```python
from build123d import *

# Parameters (mm, degrees)
BOSS_EXTRUDE2_DEPTH = 57.15
BOSS_EXTRUDE3_DEPTH = 44
CUT_EXTRUDE1_DEPTH  = 44
FILLET1_R           = 10
SKETCH6_W           = 120
SKETCH6_H           = 460.0000000000001
BOSS_EXTRUDE4_DEPTH = 10


with BuildPart() as part:
    # Sketch1 → Boss-Extrude2 (new body)
    with BuildSketch(Plane.XY):
        Polygon((0, 0), (0, 446.2018372120283), (-775, 446.2018372120282), (-774.9999999999995, -1585.7981627879717), (0, -1585.7981627879717), align=None)
    extrude(amount=BOSS_EXTRUDE2_DEPTH)

    # Sketch4 → Boss-Extrude3 (add)
    with BuildSketch(Plane.XY.offset(57.15)):
        Polygon((-79.99999999999993, -603.7981627879718), (-49.999999999999936, -603.7981627879718), (-49.999999999999915, -785.7981627879718), (-79.9999999999999, -785.7981627879718), align=None)
    extrude(amount=BOSS_EXTRUDE3_DEPTH)

    # Sketch5 → Cut-Extrude1 (cut)
    with BuildSketch(Plane.ZY.offset(80.00000000000003)):
        Polygon((83.14999999999999, -624.7981627879717), (57.150000000000006, -624.7981627879717), (57.15, -764.7981627879717), (83.15, -764.7981627879717), align=None)
    extrude(amount=-CUT_EXTRUDE1_DEPTH, mode=Mode.SUBTRACT)

    # Fillet1
    # the kernel refuses this fillet: 10 mm, written as the material it takes off along each edge
    with BuildSketch(Plane(origin=(-69.99999999999993, -613.7981627879718, 91.15), x_dir=(-1, -1.6e-16, 0), z_dir=(0, 1, 0))) as fillet1_piece_1_section:
        Polygon((0, 0), (FILLET1_R, 0), (FILLET1_R, FILLET1_R), (0, FILLET1_R), align=None)
    fillet1_piece_1 = extrude(amount=FILLET1_R, mode=Mode.PRIVATE)
    fillet1_piece_1 = fillet1_piece_1 - Plane(origin=(-69.99999999999993, -613.7981627879718, 91.15), x_dir=(0.7071067811865475, 0, -0.7071067811865475), z_dir=(0, 1, 0)) * Sphere(FILLET1_R, mode=Mode.PRIVATE)
    add(fillet1_piece_1, mode=Mode.SUBTRACT)
    with BuildSketch(Plane(origin=(-69.9999999999999, -775.7981627879718, 91.15), x_dir=(0, 0, 1), z_dir=(-1, -1.6e-16, 0))) as fillet1_piece_2_section:
        Polygon((0, 0), (FILLET1_R, 0), (FILLET1_R, -FILLET1_R), (0, -FILLET1_R), align=None)
    fillet1_piece_2 = extrude(amount=FILLET1_R, mode=Mode.PRIVATE)
    fillet1_piece_2 = fillet1_piece_2 - Plane(origin=(-69.9999999999999, -775.7981627879718, 91.15), x_dir=(0, 0.7071067811865475, -0.7071067811865475), z_dir=(-1, -1.6e-16, 0)) * Sphere(FILLET1_R, mode=Mode.PRIVATE)
    add(fillet1_piece_2, mode=Mode.SUBTRACT)
    with BuildSketch(Plane(origin=(-49.999999999999915, -785.7981627879718, 57.15), x_dir=(-1, 0, 0), z_dir=(0, 0, 1))) as fillet1_piece_3:
        with BuildLine():
            CenterArc((FILLET1_R, -FILLET1_R), FILLET1_R, 90, 90)
            Line((0, -FILLET1_R), (0, 0))
            Line((0, 0), (FILLET1_R, 0))
        make_face()
    extrude(amount=69, mode=Mode.SUBTRACT)
    with BuildSketch(Plane(origin=(-49.999999999999936, -603.7981627879718, 57.15), x_dir=(0, -1, 0), z_dir=(0, 0, 1))) as fillet1_piece_4:
        with BuildLine():
            CenterArc((FILLET1_R, -FILLET1_R), FILLET1_R, 90, 90)
            Line((0, -FILLET1_R), (0, 0))
            Line((0, 0), (FILLET1_R, 0))
        make_face()
    extrude(amount=69, mode=Mode.SUBTRACT)
    with BuildSketch(Plane(origin=(-79.99999999999993, -603.7981627879718, 57.15), x_dir=(1, 0, 0), z_dir=(0, 0, 1))) as fillet1_piece_5:
        with BuildLine():
            CenterArc((FILLET1_R, -FILLET1_R), FILLET1_R, 90, 90)
            Line((0, -FILLET1_R), (0, 0))
            Line((0, 0), (FILLET1_R, 0))
        make_face()
    extrude(amount=34.00000000000001, mode=Mode.SUBTRACT)
    with BuildSketch(Plane(origin=(-79.9999999999999, -785.7981627879718, 57.15), x_dir=(1, 0, 0), z_dir=(0, 0, 1))) as fillet1_piece_6:
        with BuildLine():
            CenterArc((FILLET1_R, FILLET1_R), FILLET1_R, 180, 90)
            Line((0, FILLET1_R), (0, 0))
            Line((0, 0), (FILLET1_R, 0))
        make_face()
    extrude(amount=34.00000000000001, mode=Mode.SUBTRACT)
    with BuildSketch(Plane(origin=(-69.99999999999993, -603.7981627879718, 101.15), x_dir=(0, 0, -1), z_dir=(1, 0, 0))) as fillet1_piece_7:
        with BuildLine():
            CenterArc((FILLET1_R, -FILLET1_R), FILLET1_R, 90, 90)
            Line((0, -FILLET1_R), (0, 0))
            Line((0, 0), (FILLET1_R, 0))
        make_face()
    extrude(amount=44.99999999999999, mode=Mode.SUBTRACT)
    with BuildSketch(Plane(origin=(-79.9999999999999, -775.7981627879718, 101.15), x_dir=(0, 0, -1), z_dir=(-1.6e-16, 1, 0))) as fillet1_piece_8:
        with BuildLine():
            CenterArc((FILLET1_R, -FILLET1_R), FILLET1_R, 90, 90)
            Line((0, -FILLET1_R), (0, 0))
            Line((0, 0), (FILLET1_R, 0))
        make_face()
    extrude(amount=162, mode=Mode.SUBTRACT)
    with BuildSketch(Plane(origin=(-24.999999999999915, -785.7981627879718, 101.15), x_dir=(0, 0, -1), z_dir=(-1, 0, 0))) as fillet1_piece_9:
        with BuildLine():
            CenterArc((FILLET1_R, -FILLET1_R), FILLET1_R, 90, 90)
            Line((0, -FILLET1_R), (0, 0))
            Line((0, 0), (FILLET1_R, 0))
        make_face()
    extrude(amount=44.999999999999986, mode=Mode.SUBTRACT)
    with BuildSketch(Plane(origin=(-79.99999999999991, -764.7981627879717, 57.15000000000002), x_dir=(1.42e-15, -1, 0), z_dir=(0, 0, 1))) as fillet1_piece_10:
        with BuildLine():
            CenterArc((FILLET1_R, FILLET1_R), FILLET1_R, 180, 89.99999999999989)
            Line((1.421e-14, FILLET1_R), (0, 0))
            Line((0, 0), (FILLET1_R, 0))
        make_face()
    extrude(amount=25.999999999999986, mode=Mode.SUBTRACT)
    with BuildSketch(Plane(origin=(-79.99999999999993, -624.7981627879717, 83.14999999999999), x_dir=(0, 1, 0), z_dir=(0, 0, -1))) as fillet1_piece_11:
        with BuildLine():
            CenterArc((FILLET1_R, FILLET1_R), FILLET1_R, 180, 90)
            Line((0, FILLET1_R), (0, 0))
            Line((0, 0), (FILLET1_R, 0))
        make_face()
    extrude(amount=25.999999999999986, mode=Mode.SUBTRACT)
    with BuildSketch(Plane(origin=(-79.99999999999991, -764.7981627879717, 83.15), x_dir=(1.42e-15, 1e-16, 1), z_dir=(-1.5e-16, 1, -1e-16))) as fillet1_piece_12:
        with BuildLine():
            CenterArc((FILLET1_R, FILLET1_R), FILLET1_R, 180, 89.99999999999989)
            Line((1.421e-14, FILLET1_R), (0, 0))
            Line((0, 0), (FILLET1_R, 0))
        make_face()
    extrude(amount=140, mode=Mode.SUBTRACT)
    with BuildSketch(Plane(origin=(-49.999999999999915, -764.7981627879717, 83.15), x_dir=(0, -1, 0), z_dir=(0, 0, -1))) as fillet1_piece_13:
        with BuildLine():
            CenterArc((FILLET1_R, FILLET1_R), FILLET1_R, 180, 90)
            Line((0, FILLET1_R), (0, 0))
            Line((0, 0), (FILLET1_R, 0))
        make_face()
    extrude(amount=26, mode=Mode.SUBTRACT)
    with BuildSketch(Plane(origin=(-49.999999999999936, -624.7981627879717, 57.150000000000006), x_dir=(0, 1, 0), z_dir=(0, 0, 1))) as fillet1_piece_14:
        with BuildLine():
            CenterArc((FILLET1_R, FILLET1_R), FILLET1_R, 180.00000000000003, 90)
            Line((0, FILLET1_R), (0, 0))
            Line((0, 0), (FILLET1_R, 0))
        make_face()
    extrude(amount=25.999999999999986, mode=Mode.SUBTRACT)
    with BuildSketch(Plane(origin=(-49.999999999999936, -624.7981627879717, 83.15), x_dir=(0, 1e-16, 1), z_dir=(1.2e-16, -1, 1e-16))) as fillet1_piece_15:
        with BuildLine():
            CenterArc((FILLET1_R, FILLET1_R), FILLET1_R, 180, 90)
            Line((0, FILLET1_R), (0, 0))
            Line((0, 0), (FILLET1_R, 0))
        make_face()
    extrude(amount=140, mode=Mode.SUBTRACT)
    with BuildSketch(Plane(origin=(-79.99999999999991, -764.7981627879717, 57.15000000000002), x_dir=(1.42e-15, -1, 0), z_dir=(0, 0, 1))) as fillet1_piece_16a_section:
        with BuildLine():
            CenterArc((FILLET1_R, FILLET1_R), FILLET1_R, 180, 89.99999999999989)
            Line((1.421e-14, FILLET1_R), (0, 0))
            Line((0, 0), (FILLET1_R, 0))
        make_face()
    fillet1_piece_16a = extrude(amount=50.999999999999986, mode=Mode.PRIVATE)
    fillet1_piece_16a = split(fillet1_piece_16a, bisect_by=Plane(origin=(-77.7360488573316, -767.0621139306398, 83.15), z_dir=(0, 1e-16, 1)), keep=Keep.TOP, mode=Mode.PRIVATE)
    with BuildSketch(Plane(origin=(-79.9999999999999, -789.7981627879717, 83.15), x_dir=(0, 1e-16, 1), z_dir=(-1.5e-16, 1, -1e-16))) as fillet1_piece_16b_section:
        with BuildLine():
            CenterArc((FILLET1_R, FILLET1_R), FILLET1_R, 180, 90)
            Line((0, FILLET1_R), (0, 0))
            Line((0, 0), (FILLET1_R, 0))
        make_face()
    fillet1_piece_16b = extrude(amount=165, mode=Mode.PRIVATE)
    fillet1_piece_16b = split(fillet1_piece_16b, bisect_by=Plane(origin=(-77.73604885733165, -764.7981627879717, 85.41395114266827), z_dir=(1.5e-16, -1, 0)), keep=Keep.TOP, mode=Mode.PRIVATE)
    fillet1_piece_16 = fillet1_piece_16a & fillet1_piece_16b
    add(fillet1_piece_16, mode=Mode.SUBTRACT)
    with BuildSketch(Plane(origin=(-79.99999999999991, -764.7981627879717, 83.15), x_dir=(1.42e-15, 1e-16, 1), z_dir=(-1.5e-16, 1, -1e-16))) as fillet1_piece_17a_section:
        with BuildLine():
            CenterArc((FILLET1_R, FILLET1_R), FILLET1_R, 180, 89.99999999999989)
            Line((1.421e-14, FILLET1_R), (0, 0))
            Line((0, 0), (FILLET1_R, 0))
        make_face()
    fillet1_piece_17a = extrude(amount=165, mode=Mode.PRIVATE)
    fillet1_piece_17a = split(fillet1_piece_17a, bisect_by=Plane(origin=(-77.73604885733167, -624.7981627879717, 85.41395114266825), z_dir=(-1.5e-16, 1, 0)), keep=Keep.TOP, mode=Mode.PRIVATE)
    with BuildSketch(Plane(origin=(-79.99999999999993, -624.7981627879717, 108.14999999999998), x_dir=(0, 1, 0), z_dir=(0, 0, -1))) as fillet1_piece_17b_section:
        with BuildLine():
            CenterArc((FILLET1_R, FILLET1_R), FILLET1_R, 180, 90)
            Line((0, FILLET1_R), (0, 0))
            Line((0, 0), (FILLET1_R, 0))
        make_face()
    fillet1_piece_17b = extrude(amount=50.999999999999986, mode=Mode.PRIVATE)
    fillet1_piece_17b = split(fillet1_piece_17b, bisect_by=Plane(origin=(-77.73604885733164, -622.5342116453035, 83.14999999999999), z_dir=(0, 1e-16, 1)), keep=Keep.TOP, mode=Mode.PRIVATE)
    fillet1_piece_17 = fillet1_piece_17a & fillet1_piece_17b
    add(fillet1_piece_17, mode=Mode.SUBTRACT)
    with BuildSketch(Plane(origin=(-49.999999999999936, -624.7981627879717, 83.15), x_dir=(0, 1e-16, 1), z_dir=(1.2e-16, -1, 1e-16))) as fillet1_piece_18a_section:
        with BuildLine():
            CenterArc((FILLET1_R, FILLET1_R), FILLET1_R, 180, 90)
            Line((0, FILLET1_R), (0, 0))
            Line((0, 0), (FILLET1_R, 0))
        make_face()
    fillet1_piece_18a = extrude(amount=165, mode=Mode.PRIVATE)
    fillet1_piece_18a = split(fillet1_piece_18a, bisect_by=Plane(origin=(-52.26395114266817, -764.7981627879717, 85.41395114266827), z_dir=(1.5e-16, -1, 0)), keep=Keep.TOP, mode=Mode.PRIVATE)
    with BuildSketch(Plane(origin=(-49.999999999999915, -764.7981627879717, 108.15), x_dir=(0, -1, 0), z_dir=(0, 0, -1))) as fillet1_piece_18b_section:
        with BuildLine():
            CenterArc((FILLET1_R, FILLET1_R), FILLET1_R, 180, 90)
            Line((0, FILLET1_R), (0, 0))
            Line((0, 0), (FILLET1_R, 0))
        make_face()
    fillet1_piece_18b = extrude(amount=51, mode=Mode.PRIVATE)
    fillet1_piece_18b = split(fillet1_piece_18b, bisect_by=Plane(origin=(-52.2639511426682, -767.0621139306397, 83.15), z_dir=(0, 1e-16, 1)), keep=Keep.TOP, mode=Mode.PRIVATE)
    fillet1_piece_18 = fillet1_piece_18a & fillet1_piece_18b
    add(fillet1_piece_18, mode=Mode.SUBTRACT)
    with BuildSketch(Plane(origin=(-49.999999999999936, -624.7981627879717, 57.150000000000006), x_dir=(0, 1, 0), z_dir=(0, 0, 1))) as fillet1_piece_19a_section:
        with BuildLine():
            CenterArc((FILLET1_R, FILLET1_R), FILLET1_R, 180.00000000000003, 90)
            Line((0, FILLET1_R), (0, 0))
            Line((0, 0), (FILLET1_R, 0))
        make_face()
    fillet1_piece_19a = extrude(amount=50.999999999999986, mode=Mode.PRIVATE)
    fillet1_piece_19a = split(fillet1_piece_19a, bisect_by=Plane(origin=(-52.26395114266823, -622.5342116453035, 83.14999999999999), z_dir=(0, 1e-16, 1)), keep=Keep.TOP, mode=Mode.PRIVATE)
    with BuildSketch(Plane(origin=(-49.999999999999936, -599.7981627879717, 83.14999999999999), x_dir=(0, 1e-16, 1), z_dir=(1.2e-16, -1, 1e-16))) as fillet1_piece_19b_section:
        with BuildLine():
            CenterArc((FILLET1_R, FILLET1_R), FILLET1_R, 179.99999999999997, 90)
            Line((0, FILLET1_R), (0, 0))
            Line((0, 0), (FILLET1_R, 0))
        make_face()
    fillet1_piece_19b = extrude(amount=165, mode=Mode.PRIVATE)
    fillet1_piece_19b = split(fillet1_piece_19b, bisect_by=Plane(origin=(-52.26395114266818, -624.7981627879717, 85.41395114266824), z_dir=(-1.5e-16, 1, 0)), keep=Keep.TOP, mode=Mode.PRIVATE)
    fillet1_piece_19 = fillet1_piece_19a & fillet1_piece_19b
    add(fillet1_piece_19, mode=Mode.SUBTRACT)

    # Sketch6 → Boss-Extrude4 (add)
    with BuildSketch(Plane(origin=(0, 0, 0), x_dir=(-1, 0, 0), z_dir=(0, 0, -1))):
        with Locations((85, -694.7981627879719)):
            Rectangle(SKETCH6_W, SKETCH6_H)
    extrude(amount=BOSS_EXTRUDE4_DEPTH)


solid = part.part
```
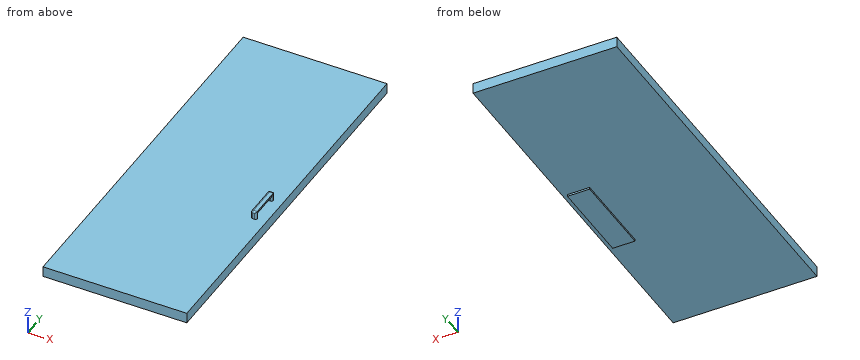
For this review, take the finished solid that the model builds, in its own axes (mm). Round coordinates to 2 decimals unless told otherwise and drop trailing zeros. Write each loop counter-clockwise with the first axis right and the second up, starting at its lowest first coordinate (ties: lowest second). Pieces come first, ordered by that corner, then holes. Notation, with made-up numbers: M 25,-29.5 L 45,-29.5 A19 ccw 45,-22.5 Z; hole C 67,5 d8. An arc over 180 degrees is marked long. One line per item, written item: value. Start each with the question number.
(1) Insertion check: pin 1 (5 mm diameter, centred on y = -768, z = -3, fed in from +X); pin 2 (6 mm diameter, centred on y = -775.5, z = 87, fed in from +X); pin 3 (11 mm diameter, centred on x = -64, z = 75.5, fed in from -Y). Each pin has a flat end and moves straight along its axis. Give the tip position at first contact, or say it passes through.
(2) We need section B-B (y = -551.5). Give the boundary of the cut face in (x, z).
(3) Wall thickness on line 1 (Z direction, x = -292, y = 227); line 2 (Z direction, x = -96, y = -521): over which ranges is each line inside the solid? List them lowest first.
(4) We need section D-D (x = -339.5). Give the boundary of the cut face in (y, z), and give its area (3 significant figures).
(5) We need section A-A (x = -100). Give the boundary of the cut face in (y, z).
(6) We need section C-C (y = -1224). Give the boundary of the cut face in (x, z), and give its area (3 significant figures).
Result:
1. pin 1: x = -25
1. pin 2: x = -50
1. pin 3: y = -785.8
2. outline: M -775,0 L -145,0 L -145,-10 L -25,-10 L -25,0 L 0,0 L 0,57.15 L -775,57.15 Z
3. line 1: 0 to 57.15
3. line 2: -10 to 57.15
4. outline: M -1585.8,0 L 446.2,0 L 446.2,57.15 L -1585.8,57.15 Z
4. area: 116,000 mm²
5. outline: M -1585.8,0 L -924.8,0 L -924.8,-10 L -464.8,-10 L -464.8,0 L 446.2,0 L 446.2,57.15 L -1585.8,57.15 Z
6. outline: M -775,0 L 0,0 L 0,57.15 L -775,57.15 Z
6. area: 44,300 mm²
